Can you work these out from the model? Positions are in its coordinate system, mm. A direction names the side the tool comes from. Give positions to 0.01 mm unless a question says otherwise; leave off trailing zeros. Loops run counter-clockwise (first coordinate to the right, second up) from the corner with the lowest first, then second, coordinate; pieces in that order, holes last. Notation, with made-up numbers: (0, 22.25) -> (30, 22.25) arc R6 cw to (30, 31.25) -> close; hole circle Ø7 at (-8.5, 44.25). An arc over 180 degrees is marked (long way). Return JSON: item names as keys, results as strings. Group by question number.
Q1. Will this pin go through, and if not, where does the flat tip stop? pin 1 (1.5 mm diameter, centred on x = -3, z = 10.5, fed in from +Y).
Q2. Suppose I cut it at C-C, the plane z = -72.5. Please give me the cut outline in (x, y).
Q3. Suppose I cut it at B-B, the plane x = 0. Please give me the cut outline in (y, z), and give its area (3 significant figures).
Q4. Thinking about a two-plate mould opening in Z: for faces 1 (the cylindrical face through (-0.65, 0.99, 69.57)), 2 (the flat face through (0, 1, -80)), 3 (the flat face through (10.5, 9, -1)), which applies, pulls with the +Z half, pulls with the -Z half, needs draft (parallel to the pull), parting line crosses it, or undercut?
Q5. Which directions (+Z, -Z, +X, -X, +Y, -Y) give clear straight access to the entire face, cutting with the end or side of a thin tool? Please do faces 4 (the flat face through (12.5, 8, -1)), 5 (the flat face through (0, 2, -1)).
Q6. I need wall thicknesses on line 1 along Z through (x, y) = (0, 0.65); line 2 along X through (y, z) = (7.5, -24); line 3 along Y through (x, z) = (3.5, 7). Which ranges of each line are inside material? Lowest first, please. Write a range as [from, to].
Q7. Suppose I cut it at A-A, the plane y = 12. Please give me the cut outline in (x, z).
Q8. Suppose I cut it at D-D, the plane z = -41. Please give me the cut outline in (x, y).
Autodesk Inventor part; units mm, degrees
ref_plane "YZ Plane" through (0, 0, 0) normal (1, 0, 0) x (0, 1, 0)
ref_plane "XZ Plane" through (0, 0, 0) normal (0, 1, 0) x (-1, 0, 0)
ref_plane "XY Plane" through (0, 0, 0) normal (0, 0, 1) x (1, 0, 0)
sketch "Szkic1" plane through (0, 0, 0) normal (0, 0, 1) x (1, 0, 0)
  line L0 (12.5, 0) -> (-12.5, 0)
  line L1 (-12.5, 0) -> (-12.5, 15)
  line L2 (12.5, 15) -> (12.5, 0)
  line L3 (-9.5, 2) -> (9.5, 2)
  line L4 (-12.5, 15) -> (-10.5, 15)
  line L5 (10.5, 15) -> (12.5, 15)
  line L6 (-10.5, 15) -> (-10.5, 3)
  line L7 (10.5, 3) -> (10.5, 15)
  arc A0 (-10.5, 3) -> (-9.5, 2) centre (-9.5, 3) ccw
  arc A1 (9.5, 2) -> (10.5, 3) centre (9.5, 3) ccw
  dimension "d2" = 25
  dimension "d3" = 15
  dimension "d5" = 1
extrude "Wyciągnięcie proste1" add sketch "Szkic1" along normal mid plane 160
sketch "Szkic2" plane through (-12.5, 0, 80) normal (0, -1, 0) x (1, 0, 0)
  circle A0 centre (12.5, -7.5) radius 3
  circle A1 centre (12.5, -152.5) radius 3
  line L0 (0, 0) -> (0, -160)
  line L1 (25, -160) -> (0, -160)
  line L2 (0, 0) -> (25, 0)
  dimension "d17" = 6
  dimension "d18" = 6
  dimension "d19" = 12.5
  dimension "d20" = 12.5
  dimension "d21" = 145
  dimension "d22" = 160
  dimension "d23" = 7.5
extrude "Wyciągnięcie proste2" cut sketch "Szkic2" against normal blind 10
equation "\"d20\" = d19"
equation "\"d23\" = -0.5 * d21 + 0.5 * d22"
properties part number "ceownik-pedal" material "Aluminium"
Ans:
{
 "1": {"pin 1": "stops at y = 2"},
 "2": {"outline": "(-12.5, 0) -> (-3, 0) -> (-3, 2) -> (-9.5, 2) arc R1 cw to (-10.5, 3) -> (-10.5, 15) -> (-12.5, 15) -> close; (3, 0) -> (12.5, 0) -> (12.5, 15) -> (10.5, 15) -> (10.5, 3) arc R1 cw to (9.5, 2) -> (3, 2) -> close"},
 "3": {"outline": "(0, -80) -> (2, -80) -> (2, -75.5) -> (0, -75.5) -> close; (0, -69.5) -> (2, -69.5) -> (2, 69.5) -> (0, 69.5) -> close; (0, 75.5) -> (2, 75.5) -> (2, 80) -> (0, 80) -> close", "area": "296 mm^2"},
 "4": {"face 1": "undercut", "face 2": "pulls with the -Z half", "face 3": "needs draft"},
 "5": {"face 4": "+Z, -Z, +X, +Y, -Y", "face 5": "+Z, -Z, +Y"},
 "6": {"line 1": "z = [-80, -75.5], [-69.5, 69.5], [75.5, 80]", "line 2": "x = [-12.5, -10.5], [10.5, 12.5]", "line 3": "y = [0, 2]"},
 "7": {"outline": "(-12.5, -80) -> (-10.5, -80) -> (-10.5, 80) -> (-12.5, 80) -> close; (10.5, -80) -> (12.5, -80) -> (12.5, 80) -> (10.5, 80) -> close"},
 "8": {"outline": "(-12.5, 0) -> (12.5, 0) -> (12.5, 15) -> (10.5, 15) -> (10.5, 3) arc R1 cw to (9.5, 2) -> (-9.5, 2) arc R1 cw to (-10.5, 3) -> (-10.5, 15) -> (-12.5, 15) -> close"}
}
